Source: CAD feature listing. Evaluate the final solid. Frame: model axes, mm. Face numbers are marked on the shaded views. A direction names the side the tool comes from. Give positions to 0.01 mm unless a question says otherwise; leave off trailing zeros. Loops run counter-clockwise (first coordinate to the right, second up) from the corner with the lowest first, then second, coordinate; pieces in that order, holes last. Notation, with made-up numbers: (40, -39.75) - (49, -39.75) arc R29 cw to (49, -14.75) - close; hole circle Ø8 at (70, -30.75). An arc over 180 degrees is marked (long way). Write each question's results on one line, items separated by ' | '. Start each with the question number.
(1) Reachability of the marked faces 1, 2, 3, 4 and 5 from +Z, -Z, +X, -X, +Y, -Y: full face, straight path, thin tool, end or side. Return the list, or none.
(2) Cut plane B-B on x = 2. Return the cut outline in (y, z).
(3) Cut plane D-D on x = -3.5. Return the cut outline in (y, z).
(4) Cut plane C-C on y = 1.5. Return the cut outline in (x, z) (3 decimals), then the cut area to 3 significant figures.
(5) Cut plane A-A on z = 6.8. Return the cut outline in (x, y) (3 decimals).
(6) Contact query for flat-ended pins moving along their axis: pin 1 (3.5 mm diameter, centred on x = 2.885, z = -6.8, fed in from -Y); pin 2 (1.6 mm diameter, centred on x = 6, y = 0.5, fed in from +Z); pin 3 (5 mm diameter, centred on x = -4, z = 26.5, fed in from -Y); pin 4 (4 mm diameter, centred on x = 3.5, y = 1.5, fed in from +Z). Output: stop coordinate, or through.
(7) Material intervals for line 1 along X through (y, z) = (1.65, 6.8) (3 decimals); line 2 along Y through (x, z) = (7.75, 7); line 3 along X through (y, z) = (3.5, 30.5) (3 decimals), sorted ascending. Write a range as [from, to].
from build123d import *

# Parameters (mm, degrees)
SKETCH1_W           = 17.77
SKETCH1_H           = 19.9
SKETCH1_R           = 1.45
BOSS_EXTRUDE1_DEPTH = 2
BOSS_EXTRUDE2_DEPTH = 10
BOSS_EXTRUDE4_DEPTH = 1.5
CHAMFER1_SIZE       = 2
CHAMFER2_SIZE       = 1.5
CHAMFER2_SIZE2      = 2.047943534
FILLET1_R           = 1.5
FILLET2_R           = 1
FILLET3_R           = 2


with BuildPart() as part:
    # Sketch1 → Boss-Extrude1 (new body)
    with BuildSketch(Plane(origin=(0, 0, 0), x_dir=(1, 0, 0), z_dir=(0, 1, 0))):
        Rectangle(SKETCH1_W, SKETCH1_H)
        with Locations(Location((2.885, 6.8, 0), (0, 0, 270))):
            Circle(SKETCH1_R, mode=Mode.SUBTRACT)
        with Locations(Location((2.885, -6.8, 0), (0, 0, 270))):
            Circle(SKETCH1_R, mode=Mode.SUBTRACT)
    extrude(amount=BOSS_EXTRUDE1_DEPTH)

    # Sketch2 → Boss-Extrude2 (add)
    with BuildSketch(Plane.ZY.offset(8.885)):
        Polygon((9.95, 2), (11.45, 2), (23.25, 4.9), (33.75, 4.9), (33.75, 2.9), (23.25, 2.9), (11.45, 0), (9.95, 0), align=None)
    extrude(amount=-BOSS_EXTRUDE2_DEPTH)

    # Sketch4 → Boss-Extrude4 (add)
    with BuildSketch(Plane.ZY.offset(8.885)):
        Polygon((33.75, 4.9), (23.25, 4.9), (11.45, 2), (11.45, 5.089270755), (22.886760378, 7.9), (33.75, 7.9), align=None)
    extrude(amount=-BOSS_EXTRUDE4_DEPTH)

    # Chamfer1
    chamfer1_edges = [part.edges().sort_by_distance(p)[0] for p in [
        (-8.135, 7.9, 33.75),
    ]]
    chamfer(chamfer1_edges, length=CHAMFER1_SIZE)

    # Chamfer2
    chamfer2_edges = [part.edges().sort_by_distance(p)[0] for p in [
        (-8.135, 5.089270755, 11.45),
    ]]
    chamfer2_side = [part.faces().sort_by_distance(p)[0] for p in [
        (-8.135, 3.544635377, 11.45),
    ]]
    chamfer(chamfer2_edges, length=CHAMFER2_SIZE, length2=CHAMFER2_SIZE2, reference=chamfer2_side[0])

    # Fillet1
    fillet1_edges = [part.edges().sort_by_distance(p)[0] for p in [
        (-8.885, 1, -9.95),
        (8.885, 1, -9.95),
        (8.885, 1, 9.95),
    ]]
    fillet(fillet1_edges, radius=FILLET1_R)

    # Fillet2
    fillet2_edges = [part.edges().sort_by_distance(p)[0] for p in [
        (1.115, 3.9, 33.75),
    ]]
    fillet(fillet2_edges, radius=FILLET2_R)

    # Fillet3
    fillet3_edges = [part.edges().sort_by_distance(p)[0] for p in [
        (1.115, 1, 9.95),
    ]]
    fillet(fillet3_edges, radius=FILLET3_R)


solid = part.part
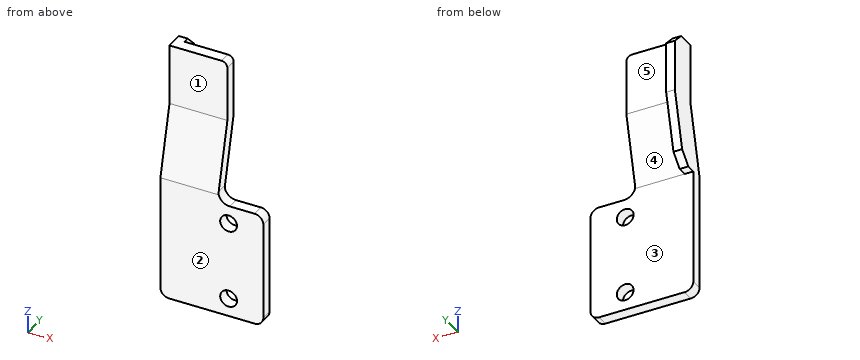
Ans:
1) face 1: +Z, +X, -X, -Y | face 2: +Z, -Z, +X, -X, -Y | face 3: -Z, +X, -X, +Y | face 4: -Z, +X, +Y | face 5: +Z, -Z, +X, +Y
2) outline: (0, -9.95) - (2, -9.95) - (2, -7.95) - (0, -7.95) - close; (0, -5.65) - (2, -5.65) - (2, 5.65) - (0, 5.65) - close; (0, 7.95) - (2, 7.95) - (2, 10.29) - (0, 10.29) - close
3) outline: (0, -9.95) - (2, -9.95) - (2, 11.45) - (4.9, 23.25) - (4.9, 33.75) - (2.9, 33.75) - (2.9, 23.25) - (0, 11.45) - close
4) outline: (-8.885, -8.45) arc R1.5 ccw to (-7.385, -9.95) - (7.385, -9.95) arc R1.5 ccw to (8.885, -8.45) - (8.885, 8.45) arc R1.5 ccw to (7.385, 9.95) - (3.115, 9.95) arc R2 cw to (1.115, 11.95) - (1.115, 17.553) - (-8.885, 17.553) - close; hole circle Ø2.9 at (2.885, -6.8); hole circle Ø2.9 at (2.885, 6.8) | area: 416 mm^2
5) outline: (-8.885, 0) - (1.435, 0) - (1.435, 2) - (-8.885, 2) - close; (4.335, 0) - (8.885, 0) - (8.885, 2) - (4.335, 2) - close
6) pin 1: y = 0 | pin 2: z = 9.95 | pin 3: y = 2.9 | pin 4: z = 10.77
7) line 1: [-8.885, 1.435], [4.335, 8.885] | line 2: [0, 2] | line 3: [-8.885, 1.115]
